Answer from the drawing. Dimensions are ordinates in mm from the lowest x, y and z of the part. A direction names the side the tool comes from. Give positions to 0.01 mm unless a question says otherwise; leave off trailing zeros. Order: outer loops, then holes, each group sorted by start corner. A loop starts at its lowest first (then second) coordinate and runs counter-clockwise, first axis right, second up. Notation, with made-up numbers: (-39.5, 51.25) - (3.5, 51.25) arc R17 ccw to (3.5, 68.25) - close; hole circle Ø8 at (43.25, 60.5). An arc over 180 degrees is marked (long way). Answer in a Markdown table with one row per item.
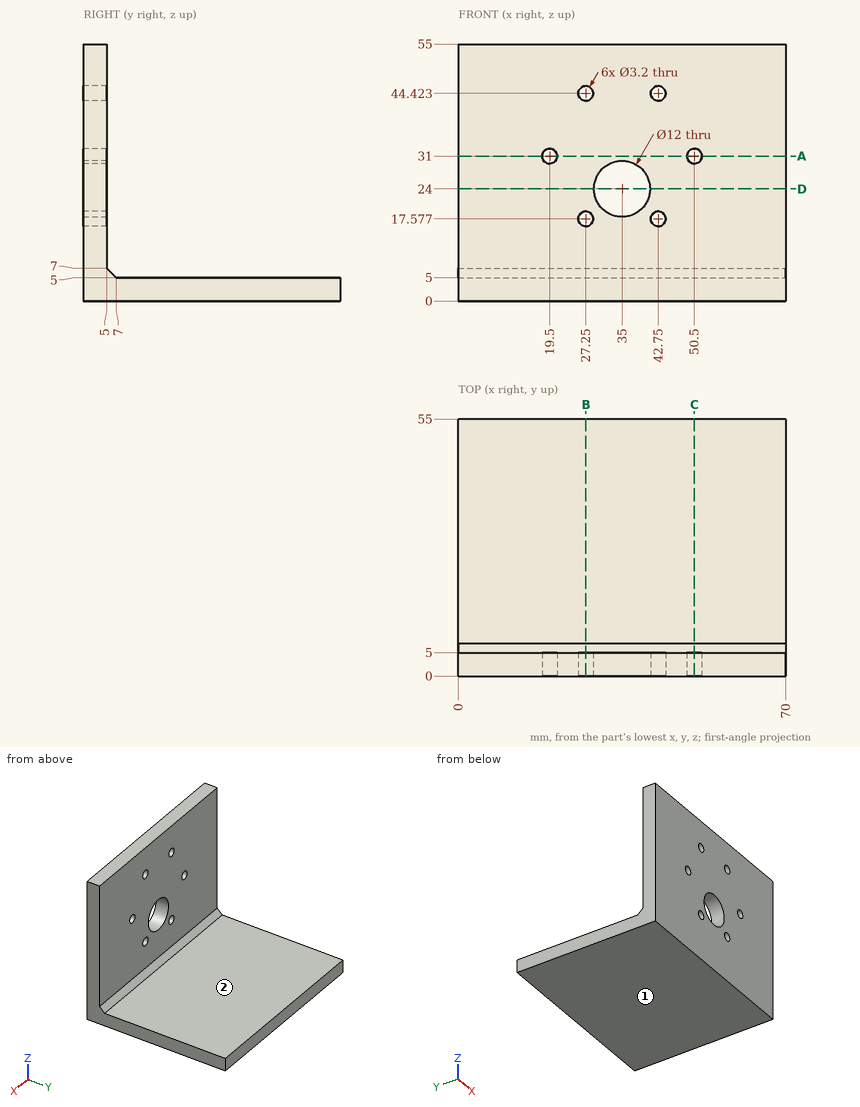
Item 1: Find section A-A on z = 31. Write down the section's boundary in (x, y).
Answer block:
| item | result |
|---|---|
| outline | (0, 0) - (17.9, 0) - (17.9, 5) - (0, 5) - close; (21.1, 0) - (48.9, 0) - (48.9, 5) - (21.1, 5) - close; (52.1, 0) - (70, 0) - (70, 5) - (52.1, 5) - close |
Item 2: Find section D-D on z = 24. Write down the section's boundary in (x, y), then the cut area to 3 significant figures.
Answer block:
| item | result |
|---|---|
| outline | (0, 0) - (29, 0) - (29, 5) - (0, 5) - close; (41, 0) - (70, 0) - (70, 5) - (41, 5) - close |
| area | 290 mm² |
Item 3: Find section C-C on x = 50.5. Write down the section's boundary in (y, z).
Answer block:
| item | result |
|---|---|
| outline | (0, 0) - (55, 0) - (55, 5) - (7, 5) - (5, 7) - (5, 29.4) - (0, 29.4) - close; (0, 32.6) - (5, 32.6) - (5, 55) - (0, 55) - close |
Item 4: Consider line 1 (X direction, y = 3.55, z = 31); line 2 (X direction, y = 3, z = 24); line 3 (Z direction, x = 50.5, y = 3.5). Determine where each line is inside the solid, lowest interval first.
Answer block:
| item | result |
|---|---|
| line 1 | 0 to 17.9, 21.1 to 48.9, 52.1 to 70 |
| line 2 | 0 to 29, 41 to 70 |
| line 3 | 0 to 29.4, 32.6 to 55 |
Item 5: Each of these flat-tipped pins is pushed along its axis until it touches: P1, Ø3, axis at x = 26, z = 46.5, coming from the +Y side; P2, Ø24, axis at x = 17.5, y = 27, coming from the +Z side. Where does it stop, or does it pass through?
Answer block:
| item | result |
|---|---|
| P1 | y = 5 |
| P2 | z = 5 |
Item 6: Which of the six approach directions +Z, -Z, +X, -X, +Y, -Y give full straight-line access (tool end or side, diameter ignored) to the marked faces 1 and 2?
Answer block:
| item | result |
|---|---|
| face 1 | -Z, +X, -X, +Y, -Y |
| face 2 | +Z, +X, -X, +Y |
Item 7: Find section B-B on x = 27.25. Write down the section's boundary in (y, z), then the cut area to 3 significant figures.
Answer block:
| item | result |
|---|---|
| outline | (0, 0) - (55, 0) - (55, 5) - (7, 5) - (5, 7) - (5, 15.98) - (0, 15.98) - close; (0, 19.18) - (5, 19.18) - (5, 42.82) - (0, 42.82) - close; (0, 46.02) - (5, 46.02) - (5, 55) - (0, 55) - close |
| area | 495 mm² |
